Verification items for the finished model (mm, model axes). A direction names the side the tool comes from. Give positions to 0.01 mm unless a question says otherwise; leave off trailing zeros. Order: outer loops, then holes, each group sorted by start corner. A loop starts at its lowest first (then second) coordinate and runs counter-clockwise, first axis right, second up.
(1) Sectioned sample at C-C on z = -1.25. Record the cut outline in (x, y), plus the area to 3 significant figures.
(2) Sectioned sample at A-A on z = -6.5. Record the cut outline in (x, y), plus the area to 3 significant figures.
(3) Sectioned sample at B-B on x = -2.5. Record the cut outline in (y, z), plus the area to 3 significant figures.
(4) Sectioned sample at D-D on z = -4.75. Count the separate pieces of the cut face and the enclosed holes in it, plus the area to 3 significant figures.
(5) Access from +Z, -Z, +X, -X, +Y, -Y to the whole of each face (thin tool, end or side, straight path). Record for faces 5 (the face through (-14.47, 0.9, -2.6)), 6 (the face through (-8, 0, -4)), 7 (the face through (-12.1, 1.11, -5.4)).
(6) Mould release check, pull along Y, two halves, no side actions. Record for faces 1 (the face through (-9, 0.71, -3)), 2 (the face through (-3, 1.11, -5)), 3 (the face through (-8, 2.54, -4)), 4 (the face through (-7.5, 1.3, 0)): pulls with the +Y half, pulls with the -Y half, needs draft (parallel to the pull), parting line crosses it, or undercut.
(7) Scan lines: L1, parallel to Y at x = -14, z = -5.5; L2, parallel to Y at x = -8.75, z = -6.5; L3, parallel to Z at x = -11.75, y = 1.05. Record each from-to range of solid material in increasing order.
(8) Gauge pin test, flat end, axial feed: pin 1 (3 mm diameter, centred on x = -12.5, z = -2, fed in from -Y). Record the tip position at first contact, or that the pin passes through.
```python
from build123d import *

# Parameters (mm, degrees)
BOSS_EXTRUDE1_DEPTH = 15.24
SKETCH2_W           = 2
SKETCH2_H           = 0.6
CUT_EXTRUDE1_DEPTH  = 5.5
SKETCH3_W           = 1
SKETCH3_H           = 1
CUT_EXTRUDE2_DEPTH  = 6
SKETCH4_W           = 2
SKETCH4_H           = 2
CUT_EXTRUDE3_DEPTH  = 0.5
CUT_EXTRUDE3_TAPER  = 45
LPATTERN1_COUNT     = 8
LPATTERN1_PITCH     = 2.54


with BuildPart() as part:
    # Sketch1 → Boss-Extrude1 (new body)
    with BuildSketch(Plane(origin=(0, 0, 0), x_dir=(0, 0, -1), z_dir=(1, 0, 0))):
        Polygon((8.5, 2.54), (0, 2.54), (0, 0), (8.5, 0), (8.5, 0.75), (7.5, 0.75), (7.5, 1.709993), (8.5, 1.709993), align=None)
    extrude(amount=-BOSS_EXTRUDE1_DEPTH)

    # Sketch2 → Cut-Extrude1 (cut)
    with BuildSketch(Plane(origin=(0, 0, -7.5), x_dir=(-1, 0, 0), z_dir=(0, 0, -1))):
        with Locations((1.27, 1.409993)):
            Rectangle(SKETCH2_W, SKETCH2_H)
    cut_extrude1 = extrude(amount=-CUT_EXTRUDE1_DEPTH, mode=Mode.SUBTRACT)

    # Sketch3 → Cut-Extrude2 (cut)
    with BuildSketch(Plane(origin=(0, 0, 0), x_dir=(-1, 0, 0), z_dir=(0, 0, -1))):
        with Locations((1.27, 1.209993)):
            Rectangle(SKETCH3_W, SKETCH3_H)
    cut_extrude2 = extrude(amount=CUT_EXTRUDE2_DEPTH, mode=Mode.SUBTRACT)

    # Sketch4 → Cut-Extrude3 (cut)
    with BuildSketch(Plane.XY):
        with Locations((-1.27, 1.209993)):
            Rectangle(SKETCH4_W, SKETCH4_H)
    cut_extrude3 = extrude(amount=-CUT_EXTRUDE3_DEPTH, taper=CUT_EXTRUDE3_TAPER, mode=Mode.SUBTRACT)

    # LPattern1: Cut-Extrude1, Cut-Extrude2, Cut-Extrude3 ×8
    with Locations(*[(-i * LPATTERN1_PITCH, 0, 0) for i in range(1, LPATTERN1_COUNT)]):
        add(cut_extrude1, mode=Mode.SUBTRACT)
        add(cut_extrude2, mode=Mode.SUBTRACT)
        add(cut_extrude3, mode=Mode.SUBTRACT)


solid = part.part
```
Ans:
1. outline: (-15.24, 0) - (0, 0) - (0, 2.54) - (-15.24, 2.54) - close; hole (-14.47, 0.71) - (-13.47, 0.71) - (-13.47, 1.71) - (-14.47, 1.71) - close; hole (-11.93, 0.71) - (-10.93, 0.71) - (-10.93, 1.71) - (-11.93, 1.71) - close; hole (-9.39, 0.71) - (-8.39, 0.71) - (-8.39, 1.71) - (-9.39, 1.71) - close; hole (-6.85, 0.71) - (-5.85, 0.71) - (-5.85, 1.71) - (-6.85, 1.71) - close; hole (-4.31, 0.71) - (-3.31, 0.71) - (-3.31, 1.71) - (-4.31, 1.71) - close; hole (-1.77, 0.71) - (-0.77, 0.71) - (-0.77, 1.71) - (-1.77, 1.71) - close
1. area: 32.7 mm2
2. outline: (-15.24, 0) - (0, 0) - (0, 2.54) - (-15.24, 2.54) - close; hole (-14.97, 1.11) - (-12.97, 1.11) - (-12.97, 1.71) - (-14.97, 1.71) - close; hole (-12.43, 1.11) - (-10.43, 1.11) - (-10.43, 1.71) - (-12.43, 1.71) - close; hole (-9.89, 1.11) - (-7.89, 1.11) - (-7.89, 1.71) - (-9.89, 1.71) - close; hole (-7.35, 1.11) - (-5.35, 1.11) - (-5.35, 1.71) - (-7.35, 1.71) - close; hole (-4.81, 1.11) - (-2.81, 1.11) - (-2.81, 1.71) - (-4.81, 1.71) - close; hole (-2.27, 1.11) - (-0.27, 1.11) - (-0.27, 1.71) - (-2.27, 1.71) - close
2. area: 31.5 mm2
3. outline: (0, -8.5) - (0.75, -8.5) - (0.75, -7.5) - (1.71, -7.5) - (1.71, -8.5) - (2.54, -8.5) - (2.54, 0) - (0, 0) - close
3. area: 20.6 mm2
4. separate pieces: 1
4. enclosed holes: 6
4. area: 29.1 mm2
5. face 5: +Z
5. face 6: +Z, -Z, +X, -X, -Y
5. face 7: -Z
6. face 1: undercut
6. face 2: undercut
6. face 3: pulls with the +Y half
6. face 4: needs draft
7. L1: y = 0 to 0.71, 1.71 to 2.54
7. L2: y = 0 to 1.11, 1.71 to 2.54
7. L3: z = -7.5 to -6
8. pin 1: stops at y = 0
